from build123d import *

# Parameters (mm, degrees)
CHAMFER_1_SIZE      = 0.5
CUT_EXTRUDE_1_DEPTH = 1.8
SKETCH_3_R          = 3
CUT_EXTRUDE_2_DEPTH = 2
SKETCH_4_W          = 1.25
SKETCH_4_H          = 0.3
CHAMFER_2_SIZE      = 0.5
SKETCH_5_W          = 0.5
SKETCH_5_H          = 0.5


with BuildPart() as part:
    # Sketch 1 → Revolve 1 (revolve)
    with BuildSketch(Plane(origin=(0, 0, 0), x_dir=(0, 0, -1), z_dir=(1, 0, 0)), mode=Mode.PRIVATE) as revolve_1_sk:
        Polygon((0, 0), (0, 16), (-5.5, 16), (-5.5, 13), (-6, 13), (-6, 13.5), (-29, 13.5), (-29, 12), (-29.5, 12), (-29.5, 12.5), (-38, 12.5), (-38, 11.95), (-39.3, 11.95), (-39.3, 12.5), (-42.5, 12.5), (-42.5, 3.5), (-43, 3.5), (-43, 4), (-55.7, 4), (-55.7, 0), align=None)
    revolve(revolve_1_sk.sketch.rotate(Axis((0, 0, 0), (0, 0, 1)), 90), axis=Axis((0, 0, 0), (0, 0, 1)))

    # Chamfer 1
    chamfer_1_edges = [part.edges().sort_by_distance(p)[0] for p in [
        (4, 0, 55.7),
    ]]
    chamfer(chamfer_1_edges, length=CHAMFER_1_SIZE)

    # Sketch 2 → Cut-Extrude 1 (cut)
    with BuildSketch(Plane(origin=(0, 4, 0), x_dir=(1, 0, 0), z_dir=(0, 1, 0))):
        with BuildLine():
            Line((-1.5, -52.5), (-1.5, -45.5))
            ThreePointArc((-1.5, -45.5), (0, -44), (1.5, -45.5))
            Line((1.5, -45.5), (1.5, -52.5))
            ThreePointArc((1.5, -52.5), (0, -54), (-1.5, -52.5))
        make_face()
    extrude(amount=-CUT_EXTRUDE_1_DEPTH, mode=Mode.SUBTRACT)

    # Sketch 3 → Cut-Extrude 2 (cut)
    with BuildSketch(Plane(origin=(0, 0, 0), x_dir=(-1, 0, 0), z_dir=(0, 0, -1))):
        Circle(SKETCH_3_R)
    extrude(amount=-CUT_EXTRUDE_2_DEPTH, mode=Mode.SUBTRACT)

    # Sketch 4 → Cut-Revolve 1 (revolve, cut)
    with BuildSketch(Plane(origin=(0, 0, 0), x_dir=(0, 0, -1), z_dir=(1, 0, 0)), mode=Mode.PRIVATE) as cut_revolve_1_sk:
        with Locations((-53.825, -3.85)):
            Rectangle(SKETCH_4_W, SKETCH_4_H)
    revolve(cut_revolve_1_sk.sketch.rotate(Axis((0, -4, 53.2), (0, 1, 0)), 180), axis=Axis((0, -4, 53.2), (0, 1, 0)), mode=Mode.SUBTRACT)

    # Chamfer 2
    chamfer_2_edges = [part.edges().sort_by_distance(p)[0] for p in [
        (3, 0, 0),
    ]]
    chamfer(chamfer_2_edges, length=CHAMFER_2_SIZE)

    # Sketch 5 → Cut-Revolve 2 (revolve, cut)
    with BuildSketch(Plane(origin=(0, 0, 0), x_dir=(0, 0, -1), z_dir=(1, 0, 0)), mode=Mode.PRIVATE) as cut_revolve_2_sk:
        with Locations((-29.75, 12.25)):
            Rectangle(SKETCH_5_W, SKETCH_5_H)
        with Locations((-6.25, 13.25)):
            Rectangle(SKETCH_5_W, SKETCH_5_H)
    revolve(cut_revolve_2_sk.sketch.rotate(Axis((0, 0, 55.7), (0, 0, -1)), 270), axis=Axis((0, 0, 55.7), (0, 0, -1)), mode=Mode.SUBTRACT)


solid = part.part
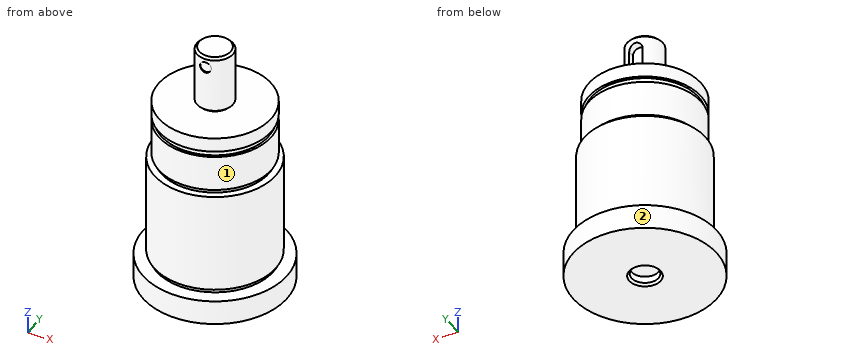
Here's how the part is built. I have some questions about the finished solid (model axes, mm). Face numbers are marked on the shaded views. A direction names the side the tool comes from. Round coordinates to 2 decimals unless told otherwise and drop trailing zeros. Loops run counter-clockwise (first coordinate to the right, second up) from the corner with the lowest first, then second, coordinate; pieces in that order, holes last. Notation, with made-up numbers: (17, 3.5) -> (35, 3.5) arc R14 cw to (35, 20.5) -> close; hole circle Ø11 at (-23, 5.5). An arc over 180 degrees is marked (long way). Write each question's results on one line, items separated by ' | '.
(1) If we section it at C-C, the plane y = -7.5: List the corners of the cut face in (x, z) for me.
Worked answers:
outline: (-14.13, 0) -> (14.13, 0) -> (14.13, 5.5) -> (10.62, 5.5) -> (10.62, 6.5) -> (11.22, 6.5) -> (11.22, 29) -> (9.37, 29) -> (9.37, 30) -> (10, 30) -> (10, 38) -> (9.3, 38) -> (9.3, 39.3) -> (10, 39.3) -> (10, 42.5) -> (-10, 42.5) -> (-10, 39.3) -> (-9.3, 39.3) -> (-9.3, 38) -> (-10, 38) -> (-10, 30) -> (-9.37, 30) -> (-9.37, 29) -> (-11.22, 29) -> (-11.22, 6.5) -> (-10.62, 6.5) -> (-10.62, 5.5) -> (-14.13, 5.5) -> close
(2) If I drill on L1, parallel to Y at x = 0, z = 1.2; L2, parallel to Z at x = 10.5, y = -9.5; L3, parallel to Z at x = -8.5, y = 1.5, over which ranges is the centre line in solid material (lowest first)?
Worked answers:
L1: -16 to -3, 3 to 16 | L2: 0 to 5.5 | L3: 0 to 42.5
(3) If we section it at D-D, the plane z = 53.2: List the corners of the cut face in (x, y) for me.
Worked answers:
outline: (-1.33, 2.2) -> (-1.33, 3.77) arc R4 ccw to (-1.25, -3.8) -> (-1.25, -3.7) -> (1.25, -3.7) -> (1.25, -3.8) arc R4 ccw to (1.33, 3.77) -> (1.33, 2.2) -> close
(4) If we section it at B-B, the plane x = -8.5: List the corners of the cut face in (y, z) for me.
Worked answers:
outline: (-13.56, 0) -> (13.56, 0) -> (13.56, 5.5) -> (9.84, 5.5) -> (9.84, 6.5) -> (10.49, 6.5) -> (10.49, 29) -> (8.47, 29) -> (8.47, 30) -> (9.17, 30) -> (9.17, 38) -> (8.4, 38) -> (8.4, 39.3) -> (9.17, 39.3) -> (9.17, 42.5) -> (-9.17, 42.5) -> (-9.17, 39.3) -> (-8.4, 39.3) -> (-8.4, 38) -> (-9.17, 38) -> (-9.17, 30) -> (-8.47, 30) -> (-8.47, 29) -> (-10.49, 29) -> (-10.49, 6.5) -> (-9.84, 6.5) -> (-9.84, 5.5) -> (-13.56, 5.5) -> close
(5) For P1, Ø1.5, axis at x = 0, z = 53.2, coming from the +Y side; P2, Ø9.5, axis at x = 0, y = 0, coming from the -Z side; P3, Ø12, axis at x = -7.5, y = -8, coming from the +Z side; P4, Ø1.2, axis at y = 3, z = 48.5, coming from the -X side, each with a flat end and sliding along its axis, tell me the tip position at first contact or that it passes through.
Worked answers:
P1: y = 2.2 | P2: z = 0 | P3: z = 42.5 | P4: x = -3.2
(6) If we section it at A-A, the plane z = 8.5: List the corners of the cut face in (x, y) for me, then the cut area to 3 significant figures.
Worked answers:
outline: circle Ø27 at (0, 0) | area: 573 mm2
(7) For the marked faces 1 and 2, which set-ups out of +Z, -Z, +X, -X, +Y, -Y let a thin tool reach every point of the face, with its end or its side?
Worked answers:
face 1: +Z | face 2: +Z, -Z
